```python
from build123d import *

# Parameters (mm, degrees)
SKICA1_W                 = 100
SKICA1_H                 = 60
VYSUNOUT1_DEPTH          = 60
ZAOBLIT1_R               = 10
SKO_EPINA1_T             = -5
SKICA2_R                 = 7.5
ODEBRAT_VYSUNUT_M2_DEPTH = 101
SKICA3_R                 = 5
VYSUNOUT2_DEPTH          = 30


with BuildPart() as part:
    # Skica1 → Vysunout1 (new body)
    with BuildSketch(Plane.XY):
        with Locations((50, 30)):
            Rectangle(SKICA1_W, SKICA1_H)
    extrude(amount=VYSUNOUT1_DEPTH)

    # Zaoblit1
    zaoblit1_edges = [part.edges().sort_by_distance(p)[0] for p in [
        (100, 30, 60),
        (0, 30, 60),
        (100, 30, 0),
        (0, 30, 0),
    ]]
    fillet(zaoblit1_edges, radius=ZAOBLIT1_R)

    # Skořepina1
    sko_epina1_openings = [part.faces().sort_by_distance(p)[0] for p in [
        (50, 60, 30),
    ]]
    offset(amount=SKO_EPINA1_T, openings=sko_epina1_openings, kind=Kind.INTERSECTION)

    # Skica2 → Odebrat vysunutím2 (cut, through all)
    with BuildSketch(Plane(origin=(100, 0, 0), x_dir=(0, 0, -1), z_dir=(1, 0, 0))):
        with Locations((-30, 40)):
            Circle(SKICA2_R)
    extrude(amount=-ODEBRAT_VYSUNUT_M2_DEPTH, mode=Mode.SUBTRACT)

    # Skica3 → Vysunout2 (add)
    with BuildSketch(Plane(origin=(0, 0, 0), x_dir=(-1, 0, 0), z_dir=(0, 0, -1))):
        with Locations((-76.959009894, 42.942278301)):
            Circle(SKICA3_R)
        with Locations((-26.264349984, 42.942278301)):
            Circle(SKICA3_R)
    extrude(amount=VYSUNOUT2_DEPTH)


solid = part.part
```
Can you work these out from the model? Positions are in its coordinate system, mm. A direction names the side the tool comes from. Round coordinates to 2 decimals unless told otherwise and drop trailing zeros. Loops run counter-clockwise (first coordinate to the right, second up) from the corner with the lowest first, then second, coordinate; pieces in that order, holes last. Notation, with made-up numbers: M 48,89 L 71,89 A37 ccw 71,127 Z; hole C -39,88.25 d4. An arc over 180 degrees is marked long. Answer as a JSON object with one key per item and string values. Group by question number.
Q1. Imagine slicing it at B-B, the plane y = 50. Please give me the cut outline in (x, z), then the cut area to 3 significant figures.
Q2. We'd pull the mould along Z, two halves only. Please class faces 3 (the flat face through (77, 43, -30)), 4 (the cylindrical face through (94, 33, 53)), 5 (the cylindrical face through (77.6, 47.9, -14.8)), 6 (the cylindrical face through (2.85, 30.42, 56.99)): +Z half, -Z half, draft (parallel to the pull), parting line (faces both ways), or undercut.
Q3. Will these pins go through, and if not, where does the flat tip stop? pin 1 (4 mm diameter, centred on x = 50.5, z = 25, fed in from -Y); pin 2 (6 mm diameter, centred on x = 40.5, y = 23.5, fed in from -Z); pin 3 (12 mm diameter, centred on y = 40, z = 30, fed in from +X); pin 4 (5 mm diameter, centred on x = 49, z = 26, fed in from +Y).
Q4. Imagine slicing it at D-D, the plane x = 38.5. Please give me the cut outline in (y, z).
Q5. Please list where these lines run through material, in increasing order: L1, parallel to X at y = 52, z = 41; L2, parallel to Z at x = 79.5, y = 47; L3, parallel to Y at x = 98, z = 30.
Q6. Imagine slicing it at A-A, the plane z = 30. Please give me the cut outline in (x, y), then the cut area to 3 significant figures.
Q7. On a 3-axis mill with a long thin cutter (end or side, diameter ignored), from which of +Z, -Z, +X, -X, +Y, -Y can I reach the whole of each face in a straight line? I mean faces 1 (the cylindrical face through (6, 33, 53)), 2 (the flat face through (49, 30, 60)). Say none if no direction works.
Findings:
{
 "1": {"outline": "M 0,10 A10 ccw 10,0 L 90,0 A10 ccw 100,10 L 100,50 A10 ccw 90,60 L 10,60 A10 ccw 0,50 Z; hole M 5,10 A5 ccw 10,5 L 90,5 A5 ccw 95,10 L 95,50 A5 ccw 90,55 L 10,55 A5 ccw 5,50 Z", "area": "1,440 mm2"},
 "2": {"face 3": "-Z half", "face 4": "undercut", "face 5": "draft", "face 6": "+Z half"},
 "3": {"pin 1": "stops at y = 0", "pin 2": "stops at z = 0", "pin 3": "passes through", "pin 4": "stops at y = 5"},
 "4": {"outline": "M 0,0 L 60,0 L 60,5 L 5,5 L 5,55 L 60,55 L 60,60 L 0,60 Z"},
 "5": {"L1": "x = 0 to 5, 95 to 100", "L2": "z = -30 to 5, 55 to 60", "L3": "y = 0 to 32.5, 47.5 to 60"},
 "6": {"outline": "M 0,0 L 100,0 L 100,32.5 L 95,32.5 L 95,5 L 5,5 L 5,32.5 L 0,32.5 Z; M 0,47.5 L 5,47.5 L 5,60 L 0,60 Z; M 95,47.5 L 100,47.5 L 100,60 L 95,60 Z", "area": "900 mm2"},
 "7": {"face 1": "+Y", "face 2": "+Z, +X, -X, +Y, -Y"}
}
